Can you work these out from the model? Positions are in its coordinate system, mm. A direction names the side the tool comes from. Give positions to 0.01 mm unless a question says otherwise; leave off trailing zeros. Loops run counter-clockwise (first coordinate to the right, second up) from the corner with the lowest first, then second, coordinate; pieces in that order, holes last. Notation, with made-up numbers: (62.5, 61) - (78.5, 61) arc R28 cw to (78.5, 92) - close; hole circle Ø8 at (-18, 13.25). An arc over 180 degrees is marked (long way). Use a Markdown table: item, result. Add a question column.
```python
from build123d import *


with BuildPart() as f1:
    # F0 (on Front) → F1 (revolve)
    with BuildSketch(Plane.XZ):
        with BuildLine():
            Line((12.5, -6.27), (12.5, -5.27))
            ThreePointArc((12.5, -5.27), (8.40016, -3.244675), (4, -2))
            ThreePointArc((4, -2), (2.236068, -0.527864), (0, 0))
            Line((0, 0), (0, -85))
            Line((0, -85), (15, -85))
            Line((15, -85), (15, -82))
            Line((15, -82), (13, -80))
            ThreePointArc((13, -80), (13.887665, -75.527781), (11.375418, -71.722876))
            Line((11.375418, -71.722876), (11.375418, -70.722876))
            ThreePointArc((11.375418, -70.722876), (10.257549, -68.761152), (8, -68.722876))
            ThreePointArc((8, -68.722876), (4.460945, -47.627558), (6, -26.292876))
            ThreePointArc((6, -26.292876), (7.822876, -25.115751), (7.5, -22.97))
            Line((7.5, -22.97), (7.5, -21.97))
            Line((7.5, -21.97), (12.5, -6.27))
        make_face()
    revolve(axis=Axis((0, 0, -42.5), (0, 0, 1)))


solid = f1.part
```
1. If we mould it in two halves opening along Z, with no side actions, what happens to faces 3 (the face through (0, 0, -85)), 4 (the face through (-7.493, 0.33, -22.463)), 5 (the face through (11.923, 3.755, -5.763))? For each: released by +Z, released by -Z, zero draft, split by the parting line, or undercut.
2. Please list where these lines run through material, in increasing order: line 1 along Z through (x, y) = (-13.5, -1); line 2 along Z through (x, y) = (11.5, -8.5); line 3 along X through (y, z) = (-2, -67). Write a range as [from, to].
3. Suppose I cut it at A-A (z = -50). List the corners of the cut face in (x, y) for me.
4. Will these pins go through, and if not, where does the flat tip stop? P1, Ø4, axis at x = -6, y = -11.5, coming from the +Z side; P2, Ø4, axis at x = 6, y = 1.5, coming from the +Z side; P3, Ø5, axis at y = -1, z = -50.5, coming from the -X side.
5. On a 3-axis mill with a long thin cutter (end or side, diameter ignored), from which of +Z, -Z, +X, -X, +Y, -Y can I reach the whole of each face in a straight line? I mean faces 1 (the face through (-8.38, 7.69, -71.22)), 2 (the face through (-14.985, 0.66, -83.479)). Say none if no direction works.
6. Suppose I cut it at B-B (z = -77). List the corners of the cut face in (x, y) for me.
Results below:
| question | item | result |
|---|---|---|
| 1 | face 3 | released by -Z |
| 1 | face 4 | undercut |
| 1 | face 5 | zero draft |
| 2 | line 1 | [-85, -80.54], [-78.99, -74.37] |
| 2 | line 2 | [-85, -81.3] |
| 2 | line 3 | [-7.24, 7.24] |
| 3 | outline | circle Ø9.21 at (0, 0) |
| 4 | P1 | z = -4.4 |
| 4 | P2 | z = -2.04 |
| 4 | P3 | x = -4.86 |
| 5 | face 1 | none |
| 5 | face 2 | +Z, -Z |
| 6 | outline | circle Ø27.98 at (0, 0) |
